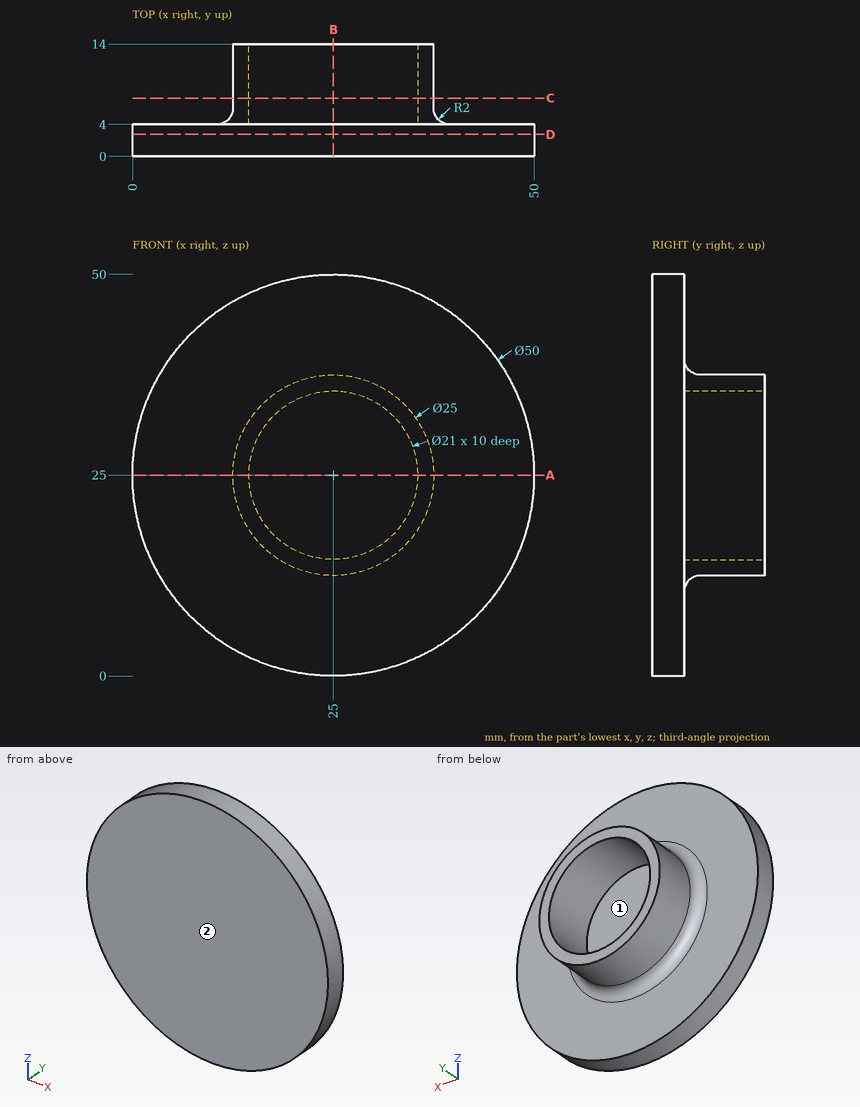
Here's the drawing with two shaded views (mm, measured from the low corner). I have some questions. A direction names the side the tool comes from. Coordinates: 2 decimals unless noted, no trailing zeros. Write each loop counter-clockwise with the first axis right and the second up, starting at its lowest first coordinate (ties: lowest second). Pieces come first, ordered by that corner, then holes. Notation, with made-up numbers: (5.25, 24.5) -> (19.25, 24.5) arc R13 ccw to (19.25, 38.5) -> close; hole circle Ø6 at (89.5, -19). An arc over 180 degrees is marked (long way). Use a Markdown table: item, result. Add a question column.
(1) If we section it at A-A, the plane z = 25: Write out the boundary of the cut face in (x, y).
(2) If we section it at D-D, the plane y = 2.75: Write out the boundary of the cut face in (x, z).
(3) If we section it at C-C, the plane y = 7.25: Write out the boundary of the cut face in (x, z).
(4) If we section it at B-B, the plane x = 25: Write out the boundary of the cut face in (y, z).
(5) For the marked faces 1 and 2, which set-ups out of +Z, -Z, +X, -X, +Y, -Y let a thin tool reach every point of the face, with its end or its side?
(6) I'm going to push flat-ended pins straight in: P1, Ø3, axis at x = 15.5, y = 2.5, coming from the +Z side; P2, Ø5, axis at y = 8, z = 30, coming from the -X side; P3, Ø5, axis at x = 27.5, y = 5.5, coming from the +Z side (3 decimals); P4, Ø1, axis at x = 38.5, y = 5.5, coming from the -Z side. Where does each tip first touch, or does it pass through?
(7) Please list where these lines run through material, in increasing order: line 1 (X direction, y = 8.75, z = 25); line 2 (Z direction, x = 30, y = 8.25).
Outcome:
| question | item | result |
|---|---|---|
| 1 | outline | (0, 0) -> (50, 0) -> (50, 4) -> (39.5, 4) arc R2 cw to (37.5, 6) -> (37.5, 14) -> (35.5, 14) -> (35.5, 4) -> (14.5, 4) -> (14.5, 14) -> (12.5, 14) -> (12.5, 6) arc R2 cw to (10.5, 4) -> (0, 4) -> close |
| 2 | outline | circle Ø50 at (25, 25) |
| 3 | outline | circle Ø25 at (25, 25); hole circle Ø21 at (25, 25) |
| 4 | outline | (0, 0) -> (4, 0) -> (4, 10.5) arc R2 cw to (6, 12.5) -> (14, 12.5) -> (14, 14.5) -> (4, 14.5) -> (4, 35.5) -> (14, 35.5) -> (14, 37.5) -> (6, 37.5) arc R2 cw to (4, 39.5) -> (4, 50) -> (0, 50) -> close |
| 5 | face 1 | +Y |
| 5 | face 2 | +Z, -Z, +X, -X, -Y |
| 6 | P1 | stops at z = 48.69 |
| 6 | P2 | stops at x = 12.75 |
| 6 | P3 | stops at z = 49.995 |
| 6 | P4 | passes through |
| 7 | line 1 | x = 12.5 to 14.5, 35.5 to 37.5 |
| 7 | line 2 | z = 13.54 to 15.77, 34.23 to 36.46 |
